Part print with two shaded views. Sizes in mm from the minimum x, y, z corner. A direction names the side the tool comes from. Round coordinates to 2 decimals unless told otherwise and drop trailing zeros. Write each loop counter-clockwise with the first axis right and the second up, starting at its lowest first coordinate (ties: lowest second). Pieces come first, ordered by that corner, then holes. Notation, with made-up numbers: (-34, -2.75) -> (-23, -2.75) arc R9 ccw to (-23, 9.25) -> close; hole circle Ø3 at (1.25, -29). An arc over 180 degrees is marked (long way). Answer in a Markdown table with one row per item.
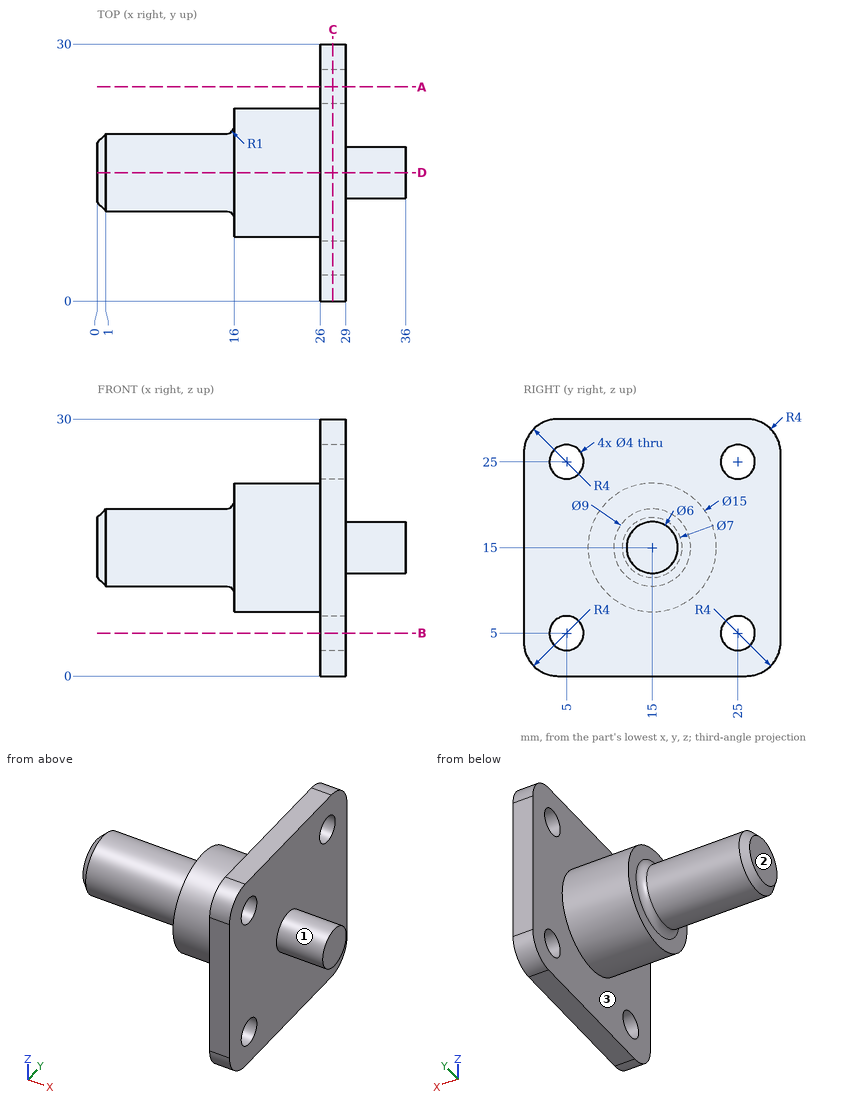
Q1. Drop flat-ended pins along their axis: P1, Ø12, axis at x = 18, y = 16, coming from the +Z side; P2, Ø6.5, axis at y = 25, z = 5, coming from the +X side; P3, Ø1, axis at x = 7.5, y = 14.5, coming from the +Z side. Give the stop position or say it passes through.
A:
| item | result |
|---|---|
| P1 | z = 22.5 |
| P2 | x = 29 |
| P3 | z = 19.5 |
Q2. Wall check: line 1 (Y direction, x = 26.7, z = 25); line 2 (X direction, y = 19.5, z = 25.75); line 3 (X direction, y = 18.5, z = 20.75). Give the ranges that are in metal, low to high. Write a range as [from, to].
A:
| item | result |
|---|---|
| line 1 | [0, 3], [7, 23], [27, 30] |
| line 2 | [26, 29] |
| line 3 | [16, 29] |
Q3. Which spindle directions (+Z, -Z, +X, -X, +Y, -Y) get a long thin tool onto all of the face, cutting with end or side? Do the marked faces 1, 2 and 3. Say none if no direction does.
A:
| item | result |
|---|---|
| face 1 | +X |
| face 2 | +Z, -Z, -X, +Y, -Y |
| face 3 | -X |
Q4. Saw through at A-A on y = 25. Write the cut outline in (x, z), plus the area to 3 significant figures.
A:
| item | result |
|---|---|
| outline | (26, 0) -> (29, 0) -> (29, 3) -> (26, 3) -> close; (26, 7) -> (29, 7) -> (29, 23) -> (26, 23) -> close; (26, 27) -> (29, 27) -> (29, 30) -> (26, 30) -> close |
| area | 66.0 mm² |
Q5. Saw through at C-C on x = 27.5. Write the cut outline in (y, z), plus the area to 3 significant figures.
A:
| item | result |
|---|---|
| outline | (0, 4) arc R4 ccw to (4, 0) -> (26, 0) arc R4 ccw to (30, 4) -> (30, 26) arc R4 ccw to (26, 30) -> (4, 30) arc R4 ccw to (0, 26) -> close; hole circle Ø4 at (5, 5); hole circle Ø4 at (5, 25); hole circle Ø4 at (25, 5); hole circle Ø4 at (25, 25) |
| area | 836 mm² |
Q6. Saw through at D-D on y = 15. Write the cut outline in (x, z).
A:
| item | result |
|---|---|
| outline | (0, 11.5) -> (1, 10.5) -> (15, 10.5) arc R1 cw to (16, 9.5) -> (16, 7.5) -> (26, 7.5) -> (26, 0) -> (29, 0) -> (29, 12) -> (36, 12) -> (36, 18) -> (29, 18) -> (29, 30) -> (26, 30) -> (26, 22.5) -> (16, 22.5) -> (16, 20.5) arc R1 cw to (15, 19.5) -> (1, 19.5) -> (0, 18.5) -> close |
